```python
from build123d import *

# Parameters (mm, degrees)
SKETCH1_R           = 25
BOSS_EXTRUDE1_DEPTH = 12.7
SKETCH2_W           = 60
SKETCH2_H           = 50
BOSS_EXTRUDE2_DEPTH = 4
SKETCH3_R           = 1.32
CUT_EXTRUDE1_DEPTH  = 17.7
SKETCH4_R           = 15
CUT_EXTRUDE2_DEPTH  = 17.7


with BuildPart() as part:
    # Sketch1 → Boss-Extrude1 (new body)
    with BuildSketch(Plane.XY):
        Circle(SKETCH1_R)
    extrude(amount=BOSS_EXTRUDE1_DEPTH)

    # Sketch2 → Boss-Extrude2 (add)
    with BuildSketch(Plane.XY.offset(12.7)):
        with Locations((-5, 0)):
            Rectangle(SKETCH2_W, SKETCH2_H)
    extrude(amount=BOSS_EXTRUDE2_DEPTH)

    # Sketch3 → Cut-Extrude1 (cut, through all)
    with BuildSketch(Plane.XY.offset(16.7)):
        with Locations((-24.985, 15.875)):
            Circle(SKETCH3_R)
        with Locations((6.765, 15.875)):
            Circle(SKETCH3_R)
        with Locations((6.765, -15.875)):
            Circle(SKETCH3_R)
        with Locations((-24.985, -15.875)):
            Circle(SKETCH3_R)
    extrude(amount=-CUT_EXTRUDE1_DEPTH, mode=Mode.SUBTRACT)

    # Sketch4 → Cut-Extrude2 (cut, through all)
    with BuildSketch(Plane.XY.offset(16.7)):
        Circle(SKETCH4_R)
    extrude(amount=-CUT_EXTRUDE2_DEPTH, mode=Mode.SUBTRACT)


solid = part.part
```
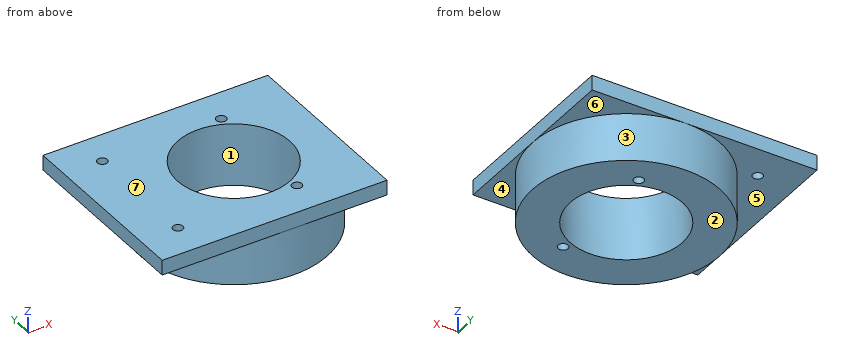
Input: part model. Units: mm. Frame: model coordinates. Face numbers are marked on the shaded views. A direction names the side the tool comes from. Coordinates: 2 decimals unless noted, no trailing zeros. Write each loop counter-clockwise with the first axis right and the second up, starting at its lowest first coordinate (ties: lowest second). Pieces come first, ordered by that corner, then holes. Notation, with made-up numbers: M 54,24 L 63,24 A16 ccw 63,53 Z; hole C 55,43 d10. An arc over 180 degrees is marked long. Use one line per item in the form item = value.
Q1. Material intervals for probe 1 along Y at (x, z) = (0, 12.5); probe 2 along X at (y, z) = (8, 8); probe 3 along Y at (x, z) = (10.5, 11.5), sorted ascending. Write a range as from..to.
Answer below:
probe_1 = -25..-15, 15..25
probe_2 = -23.69..-12.69, 12.69..23.69
probe_3 = -22.69..-10.71, 10.71..22.69
Q2. Section A-A (y = -6.5). Return loops of the section in (x, z), plus the area to 3 significant figures.
Answer below:
outline = M -35,12.7 L -24.14,12.7 L -24.14,0 L -13.52,0 L -13.52,16.7 L -35,16.7 Z; M 13.52,0 L 24.14,0 L 24.14,12.7 L 25,12.7 L 25,16.7 L 13.52,16.7 Z
area = 402 mm²
Q3. Section C-C (x = 7). Return loops of the section in (y, z), plus the area to 3 significant figures.
Answer below:
outline = M -25,12.7 L -24,12.7 L -24,0 L -17.17,0 L -17.17,16.7 L -25,16.7 Z; M -14.58,0 L -13.27,0 L -13.27,16.7 L -14.58,16.7 Z; M 13.27,0 L 14.58,0 L 14.58,16.7 L 13.27,16.7 Z; M 17.17,0 L 24,0 L 24,12.7 L 25,12.7 L 25,16.7 L 17.17,16.7 Z
area = 280 mm²
Q4. Section B-B (x = -5). Return loops of the section in (y, z).
Answer below:
outline = M -25,12.7 L -24.49,12.7 L -24.49,0 L -14.14,0 L -14.14,16.7 L -25,16.7 Z; M 14.14,0 L 24.49,0 L 24.49,12.7 L 25,12.7 L 25,16.7 L 14.14,16.7 Z
Q5. First-contact query: pin 1 (2 mm diameter, centred on y = 4.5, z = 7, fed in from -X); pin 2 (1.5 mm diameter, centred on x = -26, y = -3, fed in from -Z); pin 3 (1.6 mm diameter, centred on x = 6.765, y = 15.875, fed in from +Z); pin 4 (2 mm diameter, centred on y = 0, z = 5.5, fed in from -X). Flat tips, straight axial feed; report the tip coordinate or a pass-through.
Answer below:
pin_1 = -24.75
pin_2 = 12.7
pin_3 = through
pin_4 = -25
Q6. Draft query along X for the marked faces 1, 2 and 3. Return one class per face: released by +X, released by -X, zero draft, split by the parting line, or undercut.
Answer below:
face_1 = undercut
face_2 = zero draft
face_3 = split by the parting line
Q7. Section D-D (x = -27.5). Return loops of the section in (y, z).
Answer below:
outline = M -25,12.7 L 25,12.7 L 25,16.7 L -25,16.7 Z
Q8. Set-up query: the marked faces 4, 5, 6 and 7. Return all of +Z, -Z, +X, -X, +Y, -Y with unobstructed straight access to the full face (end or side cutting, diameter ignored); none if empty.
Answer below:
face_4 = -Z, +X, -Y
face_5 = -Z, -X
face_6 = -Z, +X, +Y
face_7 = +Z, +X, -X, +Y, -Y
